from build123d import *

# Parameters (mm, degrees)
SKETCH1_W           = 50.8
SKETCH1_H           = 76.2
BOSS_EXTRUDE1_DEPTH = 25.4
SKETCH2_R           = 1.5875
CUT_EXTRUDE1_DEPTH  = 96.038097624
SKETCH3_W           = 50.8
SKETCH3_H           = 25.4
BOSS_EXTRUDE2_DEPTH = 8.1026


with BuildPart() as part:
    # Sketch1 → Boss-Extrude1 (new body)
    with BuildSketch(Plane(origin=(0, 0, 0), x_dir=(1, 0, 0), z_dir=(0, 1, 0))):
        with Locations((25.4, 38.1)):
            Rectangle(SKETCH1_W, SKETCH1_H)
    extrude(amount=BOSS_EXTRUDE1_DEPTH)

    # Sketch2 → Cut-Extrude1 (cut, through all)
    with BuildSketch(Plane(origin=(0, 25.4, 0), x_dir=(1, 0, 0), z_dir=(0, 1, 0))):
        with Locations(Location((44.45, 60.325, 0), (0, 0, 270))):
            Circle(SKETCH2_R)
        with Locations(Location((44.45, 15.875, 0), (0, 0, 270))):
            Circle(SKETCH2_R)
    extrude(amount=-CUT_EXTRUDE1_DEPTH, mode=Mode.SUBTRACT)

    # Sketch3 → Boss-Extrude2 (add)
    with BuildSketch(Plane.XY.offset(-76.2)):
        with Locations((25.4, 12.7)):
            Rectangle(SKETCH3_W, SKETCH3_H)
    extrude(amount=-BOSS_EXTRUDE2_DEPTH)


solid = part.part
Can you work these out from the model? Positions are in its coordinate system, mm. Coordinates: 2 decimals unless noted, no trailing zeros. Write each loop counter-clockwise with the first axis right and the second up, starting at its lowest first coordinate (ties: lowest second). Pieces come first, ordered by that corner, then holes. Notation, with made-up numbers: (50.25, 44.5) - (79.25, 44.5) arc R21 cw to (79.25, 83.5) - close; hole circle Ø8 at (-35, 3.25). An arc over 180 degrees is marked (long way). Return JSON: item names as keys, results as strings. Group by question number.
Item 1: We'd pull the mould along X, two halves only. Please class faces 1 (the face through (0, 13, -42)), 2 (the face through (42.9, 12.88, -60.67)), 3 (the face through (42.9, 12.88, -16.22)), 4 (the face through (25, 0, -42)): pulls with the +X half, pulls with the -X half, needs draft (parallel to the pull), parting line crosses it, or undercut.
Item 2: If we section it at A-A (x = 44.45): Write out the boundary of the cut face in (y, z), then the cut area to 3 significant figures.
Item 3: Please list where this line runs through material, in increasing order: probe 1 along X at (y, z) = (14.5, -60.5).
Return value:
{
 "1": {"face 1": "pulls with the -X half", "face 2": "undercut", "face 3": "undercut", "face 4": "needs draft"},
 "2": {"outline": "(0, -84.3) - (25.4, -84.3) - (25.4, -61.91) - (0, -61.91) - close; (0, -58.74) - (25.4, -58.74) - (25.4, -17.46) - (0, -17.46) - close; (0, -14.29) - (25.4, -14.29) - (25.4, 0) - (0, 0) - close", "area": "1,980 mm^2"},
 "3": {"probe 1": "x = 0 to 42.87, 46.03 to 50.8"}
}
